Source: CAD feature listing. Evaluate the final solid. Frame: model axes, mm. Face numbers are marked on the shaded views. A direction names the side the tool comes from. Give positions to 0.01 mm unless a question says otherwise; leave off trailing zeros. Loops run counter-clockwise (first coordinate to the right, second up) from the corner with the lowest first, then second, coordinate; pieces in that order, holes last. Notation, with made-up numbers: M 8.5,4 L 62.5,4 A25 cw 62.5,31 Z; hole C 75.25,16 d7. An arc over 180 degrees is marked long. Answer in a Markdown table with one row per item.
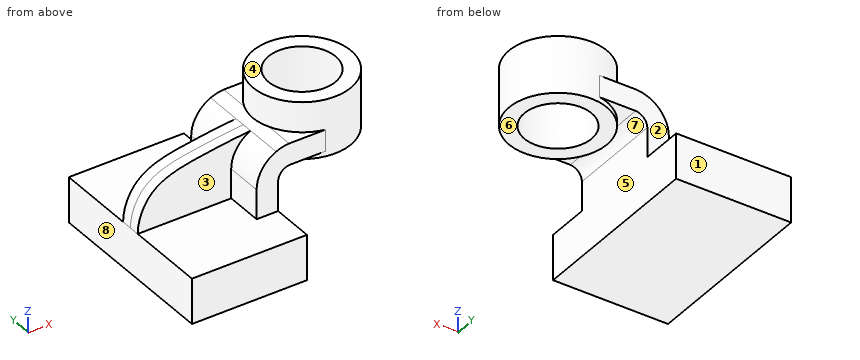
```python
from build123d import *

# Parameters (mm, degrees)
F1_DEPTH = 40
F0_W     = 16.6528351631
F0_H     = 9.5000012398
F2_DEPTH = 21.25
F3_DEPTH = 4.75
F4_W     = 21.616961807
F4_H     = 25.0849984586
F6_R     = 14.8395372195
F7_DEPTH = 61.2207443843


with BuildPart() as f1:
    # F0 (on Front) → F1 (new body, symmetric)
    with BuildSketch(Plane.XZ):
        Polygon((41.2999987602, 20), (0, 20), (0, 0), (50.8, 0), (50.8, 20), align=None)
    extrude(amount=F1_DEPTH, both=True)

    # F0 (on Front) → F2 (join, symmetric)
    with BuildSketch(Plane.XZ):
        with BuildLine():
            Line((41.2999987602, 32.9745605347), (41.2999987602, 20))
            Line((41.2999987602, 20), (50.8, 20))
            Line((50.8, 20), (50.8, 32.9745605347))
            ThreePointArc((50.8, 32.9745605347), (52.2828290923, 36.7243488741), (55.9292304386, 38.4458168319))
            Line((55.9292304386, 38.4458168319), (59.3774616718, 38.4458168319))
            Line((59.3774616718, 38.4458168319), (59.3774616718, 47.9458180717))
            Line((59.3774616718, 47.9458180717), (55.6982133685, 47.9458180717))
            ThreePointArc((55.6982133685, 47.9458180717), (52.7267880944, 47.529144235), (49.8979743732, 46.5287452266))
            ThreePointArc((49.8979743732, 46.5287452266), (43.6307882116, 41.000161872), (41.2999987602, 32.9745605347))
        make_face()
        with Locations((67.7038792534, 43.1958174518)):
            Rectangle(F0_W, F0_H)
    extrude(amount=F2_DEPTH, both=True)

    # F0 (on Front) → F3 (join, symmetric)
    with BuildSketch(Plane.XZ):
        with BuildLine():
            add(Edge.make_bspline(
                [(0, 20), (0, 26.1283031877), (5.5940842359, 39.9914167736), (28.9335310701, 43.9900934342), (44.6188528976, 46.1604342678), (49.8979743732, 46.5287452266)],
                knots=[0, 0, 0, 0, 0.31410828, 0.6650486398, 1, 1, 1, 1], degree=3))
            Line((0, 20), (41.2999987602, 20))
            Line((41.2999987602, 20), (41.2999987602, 32.9745605347))
            ThreePointArc((41.2999987602, 32.9745605347), (43.6307882116, 41.000161872), (49.8979743732, 46.5287452266))
        make_face()
    extrude(amount=F3_DEPTH, both=True)

    # F4 (on Front) → F5 (revolve)
    with BuildSketch(Plane.XZ):
        with Locations((64.9921540171, 48.677245155)):
            Rectangle(F4_W, F4_H)
    revolve(axis=Axis((75.8006349206, 0, 48.677245155), (0, 0, -1)))

    # F6 (on face) → F7 (cut, through all)
    with BuildSketch(Plane.XY.offset(61.2197443843)):
        with Locations((75.8006349206, 0)):
            Circle(F6_R)
    extrude(amount=-F7_DEPTH, mode=Mode.SUBTRACT)


solid = f1.part
```
Q1. Section query A-A (x = 64.5). Output: boundary loops of the cut face in (y, z), plus the area to 3 significant figures.
Values follow:
| item | result |
|---|---|
| outline | M -21.25,38.45 L -18.43,38.45 L -18.43,36.13 L -9.62,36.13 L -9.62,61.22 L -18.43,61.22 L -18.43,47.95 L -21.25,47.95 Z; M 9.62,36.13 L 18.43,36.13 L 18.43,38.45 L 21.25,38.45 L 21.25,47.95 L 18.43,47.95 L 18.43,61.22 L 9.62,61.22 Z |
| area | 496 mm^2 |
Q2. Section query B-B (y = -10.5). Output: boundary loops of the cut face in (x, z), plus the area to 3 significant figures.
Values follow:
| item | result |
|---|---|
| outline | M 0,0 L 50.8,0 L 50.8,32.97 A5.48 cw 55.93,38.45 L 56.91,38.45 L 56.91,36.13 L 65.31,36.13 L 65.31,61.22 L 56.91,61.22 L 56.91,47.95 L 55.7,47.95 A14.98 ccw 41.3,32.97 L 41.3,20 L 0,20 Z; M 86.29,36.13 L 94.7,36.13 L 94.7,61.22 L 86.29,61.22 Z |
| area | 1,720 mm^2 |
Q3. Contact query for flat-ended pins moving along their axis: pin 1 Ø12 at (x, y) = (26, 24) entering from +Z; pin 2 Ø10 at (y, z) = (-18.5, 11) entering from +X; pin 3 Ø14 at (x, y) = (66, -16) entering from -Z; pin 4 Ø12 at (y, z) = (-9.5, 16) entering from -X. Output: stop coordinate, or through.
Values follow:
| item | result |
|---|---|
| pin 1 | z = 20 |
| pin 2 | x = 50.8 |
| pin 3 | z = 36.13 |
| pin 4 | x = 0 |
Q4. Section query D-D (z = 13). Output: boundary loops of the cut face in (x, y), plus the area to 3 significant figures.
Values follow:
| item | result |
|---|---|
| outline | M 0,-40 L 50.8,-40 L 50.8,40 L 0,40 Z |
| area | 4,060 mm^2 |
Q5. Ray query, probe 1 along Y at (x, z) = (42.5, 21); probe 2 along Y at (x, z) = (68, 52.5); probe 3 along Z at (x, y) = (22, 30.5). Return the intervals inside material, ascending. Write a range as from..to.
Values follow:
| item | result |
|---|---|
| probe 1 | -21.25..21.25 |
| probe 2 | -20.16..-12.62, 12.62..20.16 |
| probe 3 | 0..20 |
Q6. Section query C-C (z = 56). Output: boundary loops of the cut face in (x, y), plus the area to 3 significant figures.
Values follow:
| item | result |
|---|---|
| outline | C 75.8,0 d43.23; hole C 75.8,0 d29.68 |
| area | 776 mm^2 |
Q7. Reachability of the marked faces 1, 2, 3, 4 and 5 from +Z, -Z, +X, -X, +Y, -Y: full face, straight path, thin tool, end or side. Return the list, or none.
Values follow:
| item | result |
|---|---|
| face 1 | +Z, -Z, +X, -X, +Y |
| face 2 | +Z, -X, +Y |
| face 3 | +Z, -X, -Y |
| face 4 | +Z, +X, -X, +Y, -Y |
| face 5 | -Z, +X, +Y, -Y |
Q8. Mould query, pull axis X, two halves, no side actions, for the marked faces 6, 7 and 8. Classes: +X half, -X half, draft (parallel to the pull), parting line (faces both ways), or undercut.
Values follow:
| item | result |
|---|---|
| face 6 | draft |
| face 7 | undercut |
| face 8 | -X half |
